For this review, take the finished solid that the model builds, in its own axes (mm). Face numbers are marked on the shaded views. Coordinates: 2 decimals unless noted, no trailing zeros. Order: outer loops, then holes, each group sorted by start corner. A loop starts at its lowest first (then second) coordinate and runs counter-clockwise, first axis right, second up.
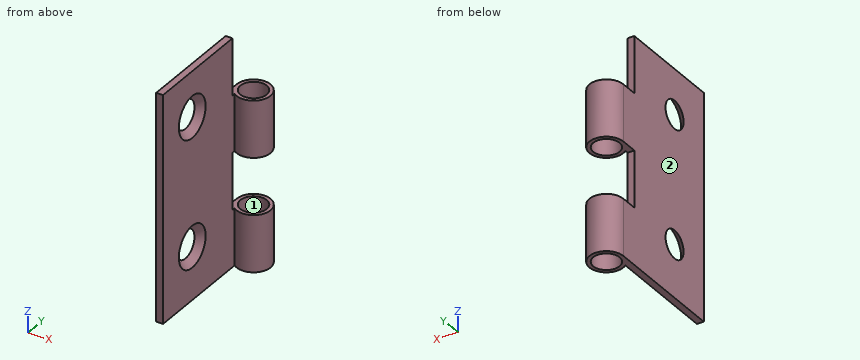
from build123d import *

# Parameters (mm, degrees)
SCHIZZO1_W                              = 0.9
SCHIZZO1_H                              = 16.5
ESTRUSIONE_SOTTILE1_DEPTH               = 15
SCHIZZO2_R                              = 2.25
SCHIZZO4_R                              = 1.75
TAGLIO_ESTRUSIONE1_DEPTH                = 36.662480284
SCHIZZO7_W                              = 7.5
SCHIZZO7_H                              = 4.5
TAGLIO_ESTRUSIONE13_DEPTH               = 10
FORO_SVASATO_PER_VITE_M2_5_1_AT_2_COUNT = 2
FORO_SVASATO_PER_VITE_M2_5_1_AT_2_PITCH = 17


with BuildPart() as part:
    # Schizzo1 → Estrusione-Sottile1 (new, symmetric)
    with BuildSketch(Plane.XY):
        with Locations((0.45, 8.25)):
            Rectangle(SCHIZZO1_W, SCHIZZO1_H)
    extrude(amount=ESTRUSIONE_SOTTILE1_DEPTH, both=True)

    # Sweep1: sweep along a curve in space
    with BuildLine() as sweep1_path:
        Line((0.9, 16.5, 15), (0.9, 16.5, -15))
    # Schizzo2 → Sweep1 (sweep)
    with BuildSketch(Plane.XY.offset(15)):
        with Locations((2.25, 16.5)):
            Circle(SCHIZZO2_R)
    sweep(path=sweep1_path.line)

    # Schizzo4 → Taglio-Estrusione1 (cut, through all)
    with BuildSketch(Plane.XY.offset(15)):
        with Locations((2.25, 16.5)):
            Circle(SCHIZZO4_R)
    extrude(amount=-TAGLIO_ESTRUSIONE1_DEPTH, mode=Mode.SUBTRACT)

    # Schizzo7 → Taglio-Estrusione13 (cut)
    with BuildSketch(Plane.ZY):
        with Locations((11.25, 16.5)):
            Rectangle(SCHIZZO7_W, SCHIZZO7_H)
        with Locations((-3.75, 16.5)):
            Rectangle(SCHIZZO7_W, SCHIZZO7_H)
    extrude(amount=-TAGLIO_ESTRUSIONE13_DEPTH, mode=Mode.SUBTRACT)

    # Schizzo8 → Foro svasato per Vite M2.5-1 (revolve, cut)
    with BuildSketch(Plane(origin=(0.9, 6, 9), x_dir=(0, 0, -1), z_dir=(0, 1, 0))):
        Polygon((0, 0), (0, 0.9), (1.45, 0.9), (1.45, 1.3), (2.75, 0), align=None)
    foro_svasato_per_vite_m2_5_1 = revolve(axis=Axis((7.25, 6, 9), (-1, 0, 0)), mode=Mode.SUBTRACT)

    # Foro svasato per Vite M2.5-1 at 2: Foro svasato per Vite M2.5-1 ×2
    with Locations(*[(0, 0, -i * FORO_SVASATO_PER_VITE_M2_5_1_AT_2_PITCH) for i in range(1, FORO_SVASATO_PER_VITE_M2_5_1_AT_2_COUNT)]):
        add(foro_svasato_per_vite_m2_5_1, mode=Mode.SUBTRACT)


solid = part.part
1. To check wall thickness, follow L1, parallel to Y at x = 2.25, z = -11.5; L2, parallel to Z at x = 0.5, y = 17.25; L3, parallel to Y at x = 0.7, z = 9.25. State the ranges of each line that lie inside material, in increasing order.
Answer below:
L1: y = 14.25 to 14.75, 18.25 to 18.75
L2: z = -15 to -7.5, 0 to 7.5
L3: y = 0 to 3.46, 8.54 to 14.25
2. Take a section at A-A, the plane z = -8. Give the boundary of the cut face in (x, y), plus the area to 3 significant figures.
Answer below:
outline: (0, 0) - (0.9, 0) - (0.9, 3.25) - (0, 4.15) - close; (0, 7.85) - (0.9, 8.75) - (0.9, 14.7) arc R2.25 ccw (long way) to (0, 16.5) - close; hole circle Ø3.5 at (2.25, 16.5)
area: 15.9 mm2
3. Take a section at D-D, the plane z = 9. Give the boundary of the cut face in (x, y), plus the area to 4 significant figures.
Answer below:
outline: (0, 0) - (0.9, 0) - (0.9, 3.25) - (0, 4.15) - close; (0, 7.85) - (0.9, 8.75) - (0.9, 14.25) - (0, 14.25) - close
area: 8.685 mm2
4. Take a section at B-B, the plane y = 6. Give the boundary of the cut face in (x, z).
Answer below:
outline: (0, -15) - (0.9, -15) - (0.9, -10.75) - (0, -9.85) - close; (0, -6.15) - (0.9, -5.25) - (0.9, 6.25) - (0, 7.15) - close; (0, 10.85) - (0.9, 11.75) - (0.9, 15) - (0, 15) - close
5. The part is to be moulded in two halves that separate along X. For the marked faces 1 and 2, say which applies: +X half, -X half, draft (parallel to the pull), parting line (faces both ways), or undercut.
Answer below:
face 1: undercut
face 2: -X half
6. Clearance check with flat-ended pins moving along their axes: pin 1 Ø8 at (y, z) = (10, -6) entering from +X; pin 2 Ø1 at (x, y) = (2, 3.5) entering from +Z; pin 3 Ø2 at (x, y) = (3.5, 16) entering from -Z; pin 4 Ø1 at (x, z) = (0.5, 9.5) entering from +Y. State where each tip first meets the part, or that it passes through.
Answer below:
pin 1: stops at x = 0.9
pin 2: passes through
pin 3: stops at z = -15
pin 4: stops at y = 14.25
7. Take a section at C-C, the plane x = 2.5. Give the boundary of the cut face in (y, z), plus the area to 3 significant figures.
Answer below:
outline: (14.26, -15) - (14.77, -15) - (14.77, -7.5) - (14.26, -7.5) - close; (14.26, 0) - (14.77, 0) - (14.77, 7.5) - (14.26, 7.5) - close; (18.23, -15) - (18.74, -15) - (18.74, -7.5) - (18.23, -7.5) - close; (18.23, 0) - (18.74, 0) - (18.74, 7.5) - (18.23, 7.5) - close
area: 15.1 mm2
